Check sheet for the modelled part. Datum: model origin and axes. Units: mm. Face numbers are marked on the shaded views. A direction names the side the tool comes from. Give positions to 0.01 mm unless a question says otherwise; leave off trailing zeros. Loops run counter-clockwise (first coordinate to the right, second up) from the corner with the lowest first, then second, coordinate; pieces in that order, holes last. Notation, with made-up numbers: M 38,-27.75 L 71,-27.75 A19 ccw 71,9.25 Z; hole C 2,4.5 d11. An arc over 180 degrees is marked long. Put each result on its own line as item: value. Start each with the question number.
```python
from build123d import *

# Parameters (mm, degrees)
SKETCH1_R           = 10
BOSS_EXTRUDE1_DEPTH = 14
SKETCH_1_R          = 6
EXTRUDE_1_DEPTH     = 15
FILLET_1_R          = 1


with BuildPart() as part:
    # Sketch1 → Boss-Extrude1 (new body, symmetric)
    with BuildSketch(Plane(origin=(0, 0, 0), x_dir=(0, 0, -1), z_dir=(1, 0, 0))):
        Circle(SKETCH1_R)
    extrude(amount=BOSS_EXTRUDE1_DEPTH, both=True)

    # 草图1 → 凸台-拉伸1 (add)
    with BuildSketch(Plane(origin=(14, 0, 0), x_dir=(0, 0, -1), z_dir=(1, 0, 0))):
        Circle(SKETCH_1_R)
    extrude_1 = extrude(amount=EXTRUDE_1_DEPTH)

    # 镜向1: 凸台-拉伸1 across plane
    add(extrude_1.mirror(Plane(origin=(0, 0, 0), x_dir=(0, 0, 1), z_dir=(1, 0, 0))))

    # 圆角1
    fillet_1_edges = [part.edges().sort_by_distance(p)[0] for p in [
        (-14, 0, 6),
        (14, 0, 6),
    ]]
    fillet(fillet_1_edges, radius=FILLET_1_R)


solid = part.part
```
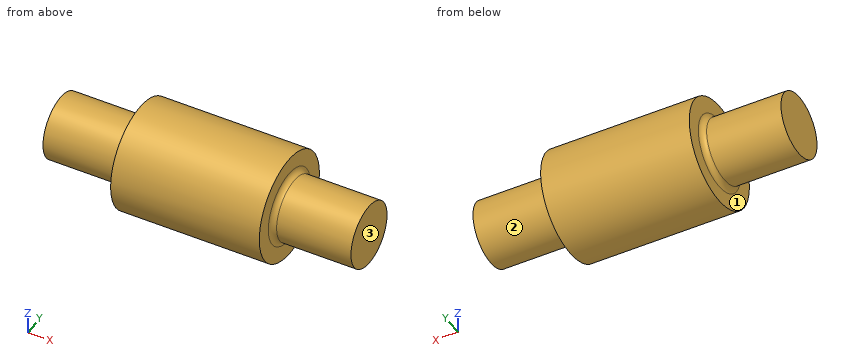
Q1. Section check C-C, the plane x = 11. Record the cut outline in (y, z).
Q2. Thickness scan on line 1 along Z through (x, y) = (8.5, 0.25); line 2 along X through (y, z) = (-0.25, -7); line 3 along Y through (x, z) = (-20.5, 0). Record the ranges inside material, lowest first. Write a range as [from, to].
Q3. Section check D-D, the plane x = -17. Record the cut outline in (y, z), then the cut area to 3 significant figures.
Q4. Section check A-A, the plane z = 0. Record the cut outline in (x, y), then the cut area to 3 significant figures.
Q5. Depth check by flat-ended pin: P1, Ø1.5, axis at x = -19, z = 3, coming from the +Y side; P2, Ø6, axis at x = -11, z = 5.5, coming from the -Y side; P3, Ø10, axis at x = 10.5, z = 6, coming from the +Y side. Enter the tip coordinate at first touch or a pass-through.
Q6. Access from +Z, -Z, +X, -X, +Y, -Y to the whole of each face (thin tool, end or side, straight path). Record for the marked faces 1, 2 and 3.
Found:
1. outline: C 0,0 d20
2. line 1: z = [-10, 10]
2. line 2: x = [-14, 14]
2. line 3: y = [-6, 6]
3. outline: C 0,0 d12
3. area: 113 mm^2
4. outline: M -29,-6 L -15,-6 A1 cw -14,-7 L -14,-10 L 14,-10 L 14,-7 A1 cw 15,-6 L 29,-6 L 29,6 L 15,6 A1 cw 14,7 L 14,10 L -14,10 L -14,7 A1 cw -15,6 L -29,6 Z
4. area: 921 mm^2
5. P1: stops at y = 5.56
5. P2: stops at y = -9.68
5. P3: stops at y = 9.95
6. face 1: -X
6. face 2: +X
6. face 3: +Z, -Z, +X, +Y, -Y
